from build123d import *

# Parameters (mm, degrees)
SKETCH1_W           = 23.454698607
SKETCH1_H           = 17.05901257
SKETCH1_R           = 2
SKETCH1_R_2         = 2.015
SKETCH1_R_3         = 2.03
SKETCH1_R_4         = 2.025
SKETCH1_R_5         = 2.035
BOSS_EXTRUDE1_DEPTH = 3


with BuildPart() as part:
    # Sketch1 → Boss-Extrude1 (new body)
    with BuildSketch(Plane(origin=(0, 0, 0), x_dir=(1, 0, 0), z_dir=(0, 1, 0))):
        with Locations((11.727349304, 8.529506285)):
            Rectangle(SKETCH1_W, SKETCH1_H)
        with Locations((4.409007026, 10.327471093)):
            Circle(SKETCH1_R, mode=Mode.SUBTRACT)
        with Locations((6.429732026, 14.216806169)):
            Circle(SKETCH1_R_2, mode=Mode.SUBTRACT)
        with Locations((16.77995554, 14.216806169)):
            Circle(SKETCH1_R_3, mode=Mode.SUBTRACT)
        with Locations((11.796158167, 14.216806169)):
            Circle(SKETCH1_R_4, mode=Mode.SUBTRACT)
        with Locations((19.665090072, 10.327471093)):
            Circle(SKETCH1_R_5, mode=Mode.SUBTRACT)
        Polygon((6.429732026, 7.459514329), (2.388282026, 7.459514329), (0.367557026, 3.959515961), (2.388282026, 0.459517593), (6.429732026, 0.459517593), (8.450457026, 3.959515961), align=None, mode=Mode.SUBTRACT)
        Polygon((13.831883167, 11.698479726), (9.760433167, 11.698479726), (7.724708167, 8.172500596), (9.760433167, 4.646521466), (13.831883167, 4.646521466), (15.867608167, 8.172500596), align=None, mode=Mode.SUBTRACT)
        Polygon((20.83640554, 7.587928947), (16.77995554, 7.587928947), (14.75173054, 4.074940198), (16.77995554, 0.561951448), (20.83640554, 0.561951448), (22.86463054, 4.074940198), align=None, mode=Mode.SUBTRACT)
    extrude(amount=BOSS_EXTRUDE1_DEPTH)


solid = part.part
The listing builds one solid part. Answer for the finished solid, in the listing's coordinates (mm). A direction names the side the tool comes from. Coordinates: 2 decimals unless noted, no trailing zeros. Order: outer loops, then holes, each group sorted by start corner. A loop starts at its lowest first (then second) coordinate and runs counter-clockwise, first axis right, second up.
Q1. Which of the six approach directions +Z, -Z, +X, -X, +Y, -Y give full straight-line access (tool end or side, diameter ignored) to faces 1 (the face through (14.864, 1.479, -9.911)), 2 (the face through (9, 0, -11))?
Q2. A cutting plane is placed at C-C, the plane y = 0.9. State how many separate pieces and enclosed holes the cut face has, and give its area (3 significant figures).
Q3. For a pull along X with two mould halves and no side action, classify faces 3 (the face through (12, 1, -17.059)), 4 (the face through (8.757, 1.479, -9.96)) as pulls with the +X half, pulls with the -X half, needs draft (parallel to the pull), parting line crosses it, or undercut.
Q4. A cutting plane is placed at A-A, the plane z = -1.5. Write down the section's boundary in (x, y), and give its area (3 significant figures).
Q5. A cutting plane is placed at D-D, the plane z = -12.75. Write down the section's boundary in (x, y).
Q6. Consider line 1 (X direction, y = 1, z = -14.25) (3 decimals); line 2 (Z direction, x = 17, y = 0.25); line 3 (Z direction, x = 3.25, y = 0.75). Determine where each line is inside the solid, lowest interval first.
Q7. A cutting plane is placed at B-B, the plane x = 3.5. Write down the section's boundary in (y, z), and give its area (3 significant figures).
Answers follow:
1. face 1: +Y, -Y
1. face 2: +Z, -Z, +X, -X, -Y
2. separate pieces: 1
2. enclosed holes: 8
2. area: 208 mm2
3. face 3: needs draft
3. face 4: undercut
4. outline: (0, 0) - (1.79, 0) - (1.79, 3) - (0, 3) - close; (7.03, 0) - (16.24, 0) - (16.24, 3) - (7.03, 3) - close; (21.38, 0) - (23.45, 0) - (23.45, 3) - (21.38, 3) - close
4. area: 39.2 mm2
5. outline: (0, 0) - (5.05, 0) - (5.05, 3) - (0, 3) - close; (7.81, 0) - (10.4, 0) - (10.4, 3) - (7.81, 3) - close; (13.19, 0) - (15.38, 0) - (15.38, 3) - (13.19, 3) - close; (18.18, 0) - (23.45, 0) - (23.45, 3) - (18.18, 3) - close
6. line 1: x = 0 to 4.415, 8.444 to 9.771, 13.821 to 14.75, 18.81 to 23.455
6. line 2: z = -17.06 to -16.23, -12.2 to -7.59, -0.56 to 0
6. line 3: z = -17.06 to -11.96, -8.7 to -7.46, -0.46 to 0
7. outline: (0, -17.06) - (3, -17.06) - (3, -12.11) - (0, -12.11) - close; (0, -8.55) - (3, -8.55) - (3, -7.46) - (0, -7.46) - close; (0, -0.46) - (3, -0.46) - (3, 0) - (0, 0) - close
7. area: 19.5 mm2
